The listing builds one solid part. Answer for the finished solid, in the listing's coordinates (mm). A direction names the side the tool comes from. Coordinates: 2 decimals unless noted, no trailing zeros. Order: outer loops, then holes, each group sorted by start corner. A loop starts at its lowest first (then second) coordinate and runs counter-clockwise, first axis right, second up. Notation, with made-up numbers: M 30,42 L 81,42 A17 cw 81,67 Z; hole C 29,26.5 d1. An arc over 180 degrees is marked long. One line per item, written item: value. Start each with the question number.
Q1. The part is cut by section B-B on z = -3.25. Give the vertices of the cut face in (x, y), then the cut area to 3 significant figures.
Q2. Straight lines are drawn through the part: line 1 along Y through (x, z) = (0, 9.7); line 2 along X through (y, z) = (120.5, 6.25). For each, find the intervals that lie inside material, in ascending order. Write a range as [from, to].
Q3. The part is cut by section C-C on y = 309. Give the vertices of the cut face in (x, z), then the cut area to 3 significant figures.
Q4. For faces 1 (the flat face through (-0.8, 450, 9.6)), 2 (the flat face through (0, 222, -9)), determine the directions among +Z, -Z, +X, -X, +Y, -Y from which every point of the face is accessible in a straight line to the end or side of a thin tool.
Q5. The part is cut by section A-A on x = 5.5. Give the vertices of the cut face in (y, z), then the cut area to 3 significant figures.
```python
from build123d import *

# Parameters (mm, degrees)
SKETCH1_W           = 20
SKETCH1_H           = 20
SKETCH1_W_2         = 18
SKETCH1_H_2         = 18
BOSS_EXTRUDE1_DEPTH = 450
SKETCH2_R           = 2.25
CUT_EXTRUDE1_DEPTH  = 451.555213043


with BuildPart() as part:
    # Sketch1 → Boss-Extrude1 (new body)
    with BuildSketch(Plane(origin=(0, 0, 0), x_dir=(1, 0, 0), z_dir=(0, 1, 0))):
        Rectangle(SKETCH1_W, SKETCH1_H)
        Rectangle(SKETCH1_W_2, SKETCH1_H_2, mode=Mode.SUBTRACT)
    extrude(amount=BOSS_EXTRUDE1_DEPTH)

    # Sketch2 → Cut-Extrude1 (cut, through all)
    with BuildSketch(Plane.XY.offset(10)):
        with Locations((0, 10)):
            Circle(SKETCH2_R)
        with BuildLine():
            Line((2.25, 440), (2.25, 390))
            ThreePointArc((2.25, 390), (0, 387.75), (-2.25, 390))
            Line((-2.25, 390), (-2.25, 440))
            ThreePointArc((-2.25, 440), (0, 442.25), (2.25, 440))
        make_face()
    extrude(amount=-CUT_EXTRUDE1_DEPTH, mode=Mode.SUBTRACT)


solid = part.part
```
Output:
1. outline: M -10,0 L -9,0 L -9,450 L -10,450 Z; M 9,0 L 10,0 L 10,450 L 9,450 Z
1. area: 900 mm^2
2. line 1: y = [0, 7.75], [12.25, 387.75], [442.25, 450]
2. line 2: x = [-10, -9], [9, 10]
3. outline: M -10,-10 L 10,-10 L 10,10 L -10,10 Z; hole M -9,-9 L 9,-9 L 9,9 L -9,9 Z
3. area: 76.0 mm^2
4. face 1: +Z, -Z, +X, -X, +Y
4. face 2: +Y, -Y
5. outline: M 0,-10 L 450,-10 L 450,-9 L 0,-9 Z; M 0,9 L 450,9 L 450,10 L 0,10 Z
5. area: 900 mm^2
